Geometry: final body of the model. Coordinates: model frame, mm. A direction names the side the tool comes from. Give positions to 0.01 mm unless a question says otherwise; leave off trailing zeros. Loops run counter-clockwise (first coordinate to the right, second up) from the corner with the lowest first, then second, coordinate; pieces in that order, holes last.
1. Material intervals for line 1 along Y through (x, z) = (6.05, 26.69) (3 decimals); line 2 along Y through (x, z) = (-2, 26.5); line 3 along X through (y, z) = (-9.5, 26), sorted ascending.
2. Section D-D, the plane z = 30. Output: boundary loops of the cut face in (x, y), then the cut area to 3 significant figures.
3. Section A-A, the plane z = 13.16. Output: boundary loops of the cut face in (x, y), then the cut area to 3 significant figures.
4. Section B-B, the plane y = -1. Output: boundary loops of the cut face in (x, z).
5. Draft query along Z for faces 1 (the face through (-10, 6, 18.16)), 2 (the face through (13.64, -9.49, 32.15)), 3 (the face through (-15, -3, 30)), 4 (the face through (13.64, -15.315, 25.653)). Return one class per face: +Z half, -Z half, draft (parallel to the pull), parting line (faces both ways), or undercut.
6. Section C-C, the plane x = 0. State how many separate pieces and enclosed holes the cut face has, then the cut area to 3 significant figures.
7. First-contact query: P1, Ø3, axis at x = 6, z = 15.5, coming from the +Y side; P2, Ø8.5, axis at x = 0.5, y = 44, coming from the +Z side; P3, Ø10, axis at x = 0, z = 8.5, coming from the -Y side; P4, Ø3, axis at x = 0, z = 30, coming from the -Y side. Flat tips, straight axial feed; report the tip coordinate or a pass-through.
8. Access query for faces 5 (the face through (-5.9, -2.54, 24.14)), 6 (the face through (14.1, 5.5, 17.3)), 7 (the face through (8, -9, 28)), 8 (the face through (15, 6, 30)), 9 (the face through (14.1, 5.46, 34.14)). Directions: +Z, -Z, +X, -X, +Y, -Y. A direction counts if a zero-diameter tool reaches every point of the face in a straight line with its end or side. Return the directions, or none.
from build123d import *

# Parameters (mm, degrees)
SKETCH_1_R          = 3.95
SKETCH_1_W          = 30
SKETCH_1_H          = 5
SKETCH_1_H_2        = 3
EXTRUDE_1_DEPTH     = 5
SKETCH_1_3_W        = 30
SKETCH_1_3_H        = 5
EXTRUDE_2_DEPTH     = 35
SKETCH_1_5_R        = 3.95
EXTRUDE_3_DEPTH     = 17.5
SKETCH_1_6_W        = 30
SKETCH_1_6_H        = 3
EXTRUDE_4_DEPTH     = 8
SKETCH_2_W          = 10
SKETCH_2_H          = 6.84
SKETCH_2_R          = 2
CUT_EXTRUDE_1_DEPTH = 16
SKETCH_2_3_W        = 10
SKETCH_2_3_H        = 10
EXTRUDE_5_DEPTH     = 13
SKETCH_2_4_W        = 10
SKETCH_2_4_H        = 10
CUT_EXTRUDE_2_DEPTH = 8
FILLET_1_R          = 3
SKETCH_3_W          = 9.92
SKETCH_3_H          = 10
CUT_EXTRUDE_4_DEPTH = 8
SKETCH_4_R          = 1.525
EXTRUDE_6_DEPTH     = 2.92


with BuildPart() as part:
    # 草图1 → 凸台-拉伸1 (new body)
    # profile 1 of 4: a face of its own
    with BuildSketch(Plane.XY):
        with BuildLine():
            ThreePointArc((-7.867496672, 46.69999866), (0, 53.25), (7.867496672, 46.69999866))
            Line((7.867496672, 46.69999866), (15, 8))
            Line((15, 8), (-15, 8))
            Line((-15, 8), (-7.867496672, 46.69999866))
        make_face()
        with Locations((0, 45.25)):
            Circle(SKETCH_1_R, mode=Mode.SUBTRACT)
    # profile 2 of 4: a face of its own
    with BuildSketch(Plane.XY):
        with Locations((0, -2.5)):
            Rectangle(SKETCH_1_W, SKETCH_1_H)
    # profile 3 of 4: a face of its own
    with BuildSketch(Plane.XY):
        with Locations((0, 5.5)):
            Rectangle(SKETCH_1_W, SKETCH_1_H)
    # profile 4 of 4: a face of its own
    with BuildSketch(Plane.XY):
        with Locations((0, 1.5)):
            Rectangle(SKETCH_1_W, SKETCH_1_H_2)
    extrude(amount=EXTRUDE_1_DEPTH)

    # 草图1<3> → 凸台-拉伸2 (add)
    with BuildSketch(Plane.XY):
        with Locations((0, 5.5)):
            Rectangle(SKETCH_1_3_W, SKETCH_1_3_H)
        with Locations((0, -2.5)):
            Rectangle(SKETCH_1_3_W, SKETCH_1_3_H)
    extrude(amount=EXTRUDE_2_DEPTH)

    # 草图1<5> → 凸台-拉伸3 (add)
    with BuildSketch(Plane.XY):
        with Locations((0, 45.25)):
            Circle(SKETCH_1_5_R)
    extrude(amount=EXTRUDE_3_DEPTH)

    # 草图1<6> → 凸台-拉伸4 (add)
    with BuildSketch(Plane.XY):
        with Locations((0, 1.5)):
            Rectangle(SKETCH_1_6_W, SKETCH_1_6_H)
    extrude(amount=EXTRUDE_4_DEPTH)

    # 草图2 → 切除-拉伸1 (cut)
    with BuildSketch(Plane(origin=(0, 8, 0), x_dir=(1, 0, 0), z_dir=(0, 1, 0))):
        with Locations((-10, -21.58)):
            Rectangle(SKETCH_2_W, SKETCH_2_H)
        with Locations((10, -21.58)):
            Rectangle(SKETCH_2_W, SKETCH_2_H)
        with Locations(Location((0, -13.16, 0), (0, 0, 270))):
            Circle(SKETCH_2_R)
        with Locations(Location((0, -30, 0), (0, 0, 270))):
            Circle(SKETCH_2_R)
    extrude(amount=-CUT_EXTRUDE_1_DEPTH, mode=Mode.SUBTRACT)

    # 草图2<3> → 凸台-拉伸5 (add)
    with BuildSketch(Plane(origin=(0, 8, 0), x_dir=(1, 0, 0), z_dir=(0, 1, 0))):
        with Locations((20, -30)):
            Rectangle(SKETCH_2_3_W, SKETCH_2_3_H)
    extrude(amount=-EXTRUDE_5_DEPTH)

    # 草图2<4> → 切除-拉伸2 (cut)
    with BuildSketch(Plane(origin=(0, 8, 0), x_dir=(1, 0, 0), z_dir=(0, 1, 0))):
        with Locations((20, -30)):
            Rectangle(SKETCH_2_4_W, SKETCH_2_4_H)
    extrude(amount=-CUT_EXTRUDE_2_DEPTH, mode=Mode.SUBTRACT)

    # 圆角1
    fillet_1_edges = [part.edges().sort_by_distance(p)[0] for p in [
        (-15, -2.5, 18.16),
        (-15, 5.5, 18.16),
        (-5, -2.5, 18.16),
        (-5, 5.5, 18.16),
        (-5, -2.5, 25),
        (-5, 5.5, 25),
        (-15, -2.5, 25),
        (-15, 5.5, 25),
        (5, -2.5, 25),
        (5, 5.5, 25),
        (5, -2.5, 18.16),
        (5, 5.5, 18.16),
        (15, -2.5, 18.16),
        (15, 5.5, 18.16),
        (15, 5.5, 35),
        (15, 5.5, 25),
        (-15, 5.5, 35),
        (-15, -2.5, 35),
    ]]
    fillet(fillet_1_edges, radius=FILLET_1_R)

    # 草图3 → 切除-拉伸4 (cut)
    with BuildSketch(Plane.XZ.offset(5)):
        with Locations((20.04, 30)):
            Rectangle(SKETCH_3_W, SKETCH_3_H)
    extrude(amount=-CUT_EXTRUDE_4_DEPTH, mode=Mode.SUBTRACT)

    # 草图4 → 凸台-拉伸6 (add)
    with BuildSketch(Plane(origin=(15.08, 0, 0), x_dir=(0, 0, -1), z_dir=(1, 0, 0))):
        with BuildLine():
            Line((-35, -5), (-29.223331883, -14.106931726))
            ThreePointArc((-29.223331883, -14.106931726), (-25.598856813, -15.294531543), (-23.738058654, -11.965170783))
            Line((-23.738058654, -11.965170783), (-25, -5))
            Line((-25, -5), (-35, -5))
        make_face()
        with Locations((-26.69, -12.5)):
            Circle(SKETCH_4_R, mode=Mode.SUBTRACT)
    extrude_6 = extrude(amount=-EXTRUDE_6_DEPTH)

    # 镜向1: 凸台-拉伸6 across plane
    add(extrude_6.mirror(Plane(origin=(10.08, 0, 0), x_dir=(0, 0, 1), z_dir=(1, 0, 0))))


solid = part.part
Answers below:
1. line 1: y = -15.5 to -14.025, -10.975 to 0, 3 to 8
1. line 2: y = -5 to 0, 3 to 8
1. line 3: x = 5.08 to 8, 12.16 to 15.08
2. outline: (-15, -5) - (-2, -5) - (-2, 0) - (-15, 0) - close; (-15, 3) - (-2, 3) - (-2, 8) - (-15, 8) - close; (2, -5) - (5.08, -5) - (5.08, -12.88) - (8, -12.88) - (8, -5) - (12.16, -5) - (12.16, -12.88) - (15.08, -12.88) - (15.08, 0) - (2, 0) - close; (2, 3) - (15, 3) - (15, 8) - (2, 8) - close
2. area: 306 mm2
3. outline: (-15, -5) - (-2, -5) - (-2, 0) - (-15, 0) - close; (-15, 3) - (-2, 3) - (-2, 8) - (-15, 8) - close; circle Ø7.9 at (0, 45.25); (2, -5) - (15, -5) - (15, 0) - (2, 0) - close; (2, 3) - (15, 3) - (15, 8) - (2, 8) - close
3. area: 309 mm2
4. outline: (-15, 0) - (15, 0) - (15, 15.16) arc R3 ccw to (12, 18.16) - (8, 18.16) arc R3 cw to (5, 21.16) - (5, 22) arc R3 cw to (8, 25) - (15.08, 25) - (15.08, 35) - (-12, 35) arc R3 ccw to (-15, 32) - (-15, 28) arc R3 ccw to (-12, 25) - (-8, 25) arc R3 cw to (-5, 22) - (-5, 21.16) arc R3 cw to (-8, 18.16) - (-12, 18.16) arc R3 ccw to (-15, 15.16) - close; hole circle Ø4 at (0, 13.16); hole circle Ø4 at (0, 30)
5. face 1: undercut
5. face 2: +Z half
5. face 3: draft
5. face 4: parting line
6. separate pieces: 5
6. enclosed holes: 0
6. area: 619 mm2
7. P1: stops at y = 8
7. P2: stops at z = 17.5
7. P3: stops at y = -5
7. P4: passes through
8. face 5: -X, +Y, -Y
8. face 6: +X, +Y, -Y
8. face 7: +Z, -Z, -Y
8. face 8: +Z, -Z, +X, +Y
8. face 9: +Z, +X, +Y
